```python
from build123d import *

# Parameters (mm, degrees)
F3_R     = 6.5
F3_R_2   = 5
F4_DEPTH = 20
F5_DEPTH = 14.3


with BuildPart() as f1:
    # F0 (on Front) → F1 (revolve)
    with BuildSketch(Plane.XZ):
        Polygon((-130.0127011951, 91.7292905117), (-133.0127011951, 91.7292905117), (-128.0937719805, 56.7292905117), (-111.2923327753, 56.7292905117), (-111.2923327753, 36.7292905117), (-108.2923327753, 36.7292905117), (-108.2923327753, 79.7292905117), (-111.2923327753, 79.7292905117), (-111.2923327753, 59.7292905117), (-125.5153944847, 59.7292905117), align=None)
    revolve(axis=Axis((-149.0423327753, 0, 54.1304184761), (0, 0, -1)))

    # F3 (on offset) → F4 (join)
    with BuildSketch(Plane.YZ.offset(-111)):
        with Locations((0, 64.2200395022)):
            Circle(F3_R)
        with Locations((0, 64.2200395022)):
            Circle(F3_R_2, mode=Mode.SUBTRACT)
    extrude(amount=F4_DEPTH)

    # F3 (on offset) → F5 (cut, symmetric)
    with BuildSketch(Plane.YZ.offset(-111)):
        with Locations((0, 64.2200395022)):
            Circle(F3_R_2)
    extrude(amount=F5_DEPTH, both=True, mode=Mode.SUBTRACT)


solid = f1.part
```
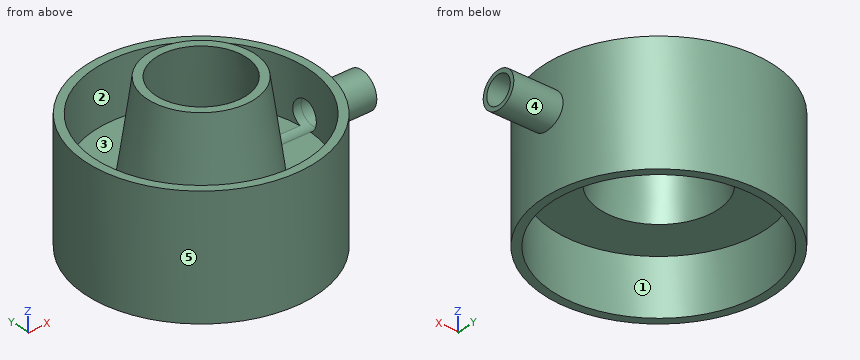
The model under review builds one solid part; all positions refer to its coordinate system, in mm. Face numbers are marked on the shaded views. A direction names the side the tool comes from. Coordinates: 2 decimals unless noted, no trailing zeros. Order: outer loops, then holes, each group sorted by start corner. A loop starts at its lowest first (then second) coordinate and runs counter-clockwise, first axis right, second up. Notation, with made-up numbers: (36.5, -39) -> (90.5, -39) arc R32 ccw to (90.5, -7) -> close; hole circle Ø10 at (-33, 25). An arc over 180 degrees is marked (long way). Answer in a Markdown table with one row per item. Add a question column.
Item 1: To check wall thickness, follow probe 1 along Y at (x, z) = (-132.5, 79.5); probe 2 along Y at (x, z) = (-163.5, 61.5); probe 3 along X at (y, z) = (14, 67.5). State the ranges of each line that lie inside material, in increasing order.
Item 2: Clearance check with flat-ended pins moving along their axes: pin 1 (5 mm diameter, centred on x = -177, y = -17, fed in from -Z); pin 2 (3 mm diameter, centred on y = -22.5, z = 83, fed in from +X); pin 3 (4 mm diameter, centred on y = 12.5, z = 57.5, fed in from +X); pin 4 (6 mm diameter, centred on y = 17.5, z = 71.5, fed in from -X). State where each tip first meets the part, or that it passes through.
Item 3: We need section D-D on z = 76. Write out the cut boundary in (x, y), plus the area to 3 significant figures.
Item 4: Mouldability with a two-part tool opening along X and no side actions: class the marked faces 3, 4 and 5 as +X half, -X half, draft (parallel to the pull), parting line (faces both ways), or undercut.
Item 5: We need section A-A on z = 68. Write out the cut boundary in (x, y), plus the area to 3 significant figures.
Item 6: Machinability: for the marked faces 1 and 2, which of the approach directions +Z, -Z, +X, -X, +Y, -Y give a long, thin tool a straight path to every point of the face, cutting with its end or side? Answer none if there is none.
Item 7: We need section C-C on y = -35. Write out the cut boundary in (x, z), plus the area to 3 significant figures.
Item 8: We need section B-B on y = 0. Write out the cut boundary in (x, z).
Final values:
| question | item | result |
|---|---|---|
| 1 | probe 1 | y = -37.24 to -33.93, -12.52 to -6.43, 6.43 to 12.52, 33.93 to 37.24 |
| 1 | probe 2 | y = -38.1 to -34.87, -18.24 to -14.22, 14.22 to 18.24, 34.87 to 38.1 |
| 1 | probe 3 | x = -187.31 to -184.1, -166.57 to -162.52, -135.56 to -131.51, -113.98 to -110.77 |
| 2 | pin 1 | stops at z = 56.73 |
| 2 | pin 2 | passes through |
| 2 | pin 3 | stops at x = -109.67 |
| 2 | pin 4 | stops at x = -187.13 |
| 3 | outline | circle Ø81.5 at (-149.04, 0); circle Ø42.48 at (-149.04, 0); hole circle Ø75.5 at (-149.04, 0); hole circle Ø36.48 at (-149.04, 0) |
| 3 | area | 1,110 mm2 |
| 4 | face 3 | undercut |
| 4 | face 4 | draft |
| 4 | face 5 | parting line |
| 5 | outline | circle Ø44.73 at (-149.04, 0); (-111.43, -3.27) arc R37.75 cw (long way) to (-111.43, 3.27) -> (-91, 3.27) -> (-91, 5.29) -> (-108.64, 5.29) arc R40.75 ccw (long way) to (-108.64, -5.29) -> (-91, -5.29) -> (-91, -3.27) -> close; hole circle Ø38.73 at (-149.04, 0) |
| 5 | area | 1,180 mm2 |
| 6 | face 1 | -Z |
| 6 | face 2 | +Z |
| 7 | outline | (-169.91, 36.73) -> (-163.19, 36.73) -> (-163.19, 56.73) -> (-134.9, 56.73) -> (-134.9, 36.73) -> (-128.17, 36.73) -> (-128.17, 79.73) -> (-134.9, 79.73) -> (-134.9, 59.73) -> (-163.19, 59.73) -> (-163.19, 79.73) -> (-169.91, 79.73) -> close |
| 7 | area | 663 mm2 |
| 8 | outline | (-189.79, 36.73) -> (-186.79, 36.73) -> (-186.79, 56.73) -> (-169.99, 56.73) -> (-165.07, 91.73) -> (-168.07, 91.73) -> (-172.57, 59.73) -> (-186.79, 59.73) -> (-186.79, 79.73) -> (-189.79, 79.73) -> close; (-133.01, 91.73) -> (-128.09, 56.73) -> (-111.29, 56.73) -> (-111.29, 36.73) -> (-108.29, 36.73) -> (-108.29, 57.72) -> (-91, 57.72) -> (-91, 59.22) -> (-125.3, 59.22) -> (-125.3, 59.73) -> (-125.52, 59.73) -> (-130.01, 91.73) -> close; (-111.29, 69.22) -> (-91, 69.22) -> (-91, 70.72) -> (-108.29, 70.72) -> (-108.29, 79.73) -> (-111.29, 79.73) -> close |
